Solid Edge part; units mm, degrees
sketch "Sketch1" plane through (0, 0, 0) normal (0, -1, 0) x (1, 0, 0)
  circle A0 centre (0, 0) radius 30.25
extrude "Protrusion1" add sketch "Sketch1" against normal blind 2
sketch "Sketch2" plane through (0, 0, 0) normal (0, -1, 0) x (1, 0, 0)
  circle A0 centre (0, 0) radius 4.5
extrude "Cutout1" cut sketch "Sketch2" against normal through all
sketch "Sketch3" plane through (0, 0, 0) normal (0, -1, 0) x (1, 0, 0)
  circle A0 centre (0, 24) radius 1.5
extrude "Cutout2" cut sketch "Sketch3" against normal through all
pattern_circular "Pattern1" count 4 over 360 about axis through (0, 0, 0) along (0, 1, 0) of "Cutout2"
Source: CAD feature listing. Evaluate the final solid. Frame: model axes, mm. Round coordinates to 2 decimals unless told otherwise and drop trailing zeros. Write each loop counter-clockwise with the first axis right and the second up, starting at its lowest first coordinate (ties: lowest second). Pieces come first, ordered by that corner, then holes. Notation, with made-up numbers: M 14.25,60 L 29.25,60 A10 cw 29.25,65 Z; hole C 68,4 d7. An arc over 180 degrees is marked long. One line per item, written item: value. Start each with the question number.
Item 1: Section query C-C (x = 24). Return the cut outline in (y, z).
Item 2: Section query B-B (z = 3). Return the cut outline in (x, y).
Item 3: Section query D-D (y = 0.85). Return the cut outline in (x, z), plus the area to 3 significant figures.
Item 4: Pin query (flat end, axial travel): pin 1 (5 mm diameter, centred on x = 0, z = 24, fed in from -Y); pin 2 (1 mm diameter, centred on y = 1.5, z = 15.5, fed in from +X). Return the tip coordinate at first contact, or that it passes through.
Item 5: Mould query, pull axis X, two halves, no side actions, for faces 1 (the flat face through (0, 2, -6)), 2 (the cylindrical face through (-0.59, 0.99, 4.46)), 3 (the cylindrical face through (-25.487, 0.986, -0.195)), 4 (the cylindrical face through (-6.56, 0.99, -29.53)). Classes: pulls with the +X half, pulls with the -X half, needs draft (parallel to the pull), parting line crosses it, or undercut.
Item 6: Section query A-A (x = 0). Return the cut outline in (y, z).
Item 7: Ray query, L1, parallel to Z at x = 0, y = 0.9; L2, parallel to Z at x = -24, y = 0.95; L3, parallel to X at y = 1.05, z = 25. Return the intervals inside material, ascending. Write a range as from..to.
Result set:
1. outline: M 0,-18.41 L 2,-18.41 L 2,-1.5 L 0,-1.5 Z; M 0,1.5 L 2,1.5 L 2,18.41 L 0,18.41 Z
2. outline: M -30.1,0 L -3.35,0 L -3.35,2 L -30.1,2 Z; M 3.35,0 L 30.1,0 L 30.1,2 L 3.35,2 Z
3. outline: C 0,0 d60.5; hole C -24,0 d3; hole C 0,0 d9; hole C 0,-24 d3; hole C 0,24 d3; hole C 24,0 d3
3. area: 2,780 mm²
4. pin 1: stops at y = 0
4. pin 2: stops at x = 26.27
5. face 1: needs draft
5. face 2: undercut
5. face 3: undercut
5. face 4: parting line crosses it
6. outline: M 0,-30.25 L 2,-30.25 L 2,-25.5 L 0,-25.5 Z; M 0,-22.5 L 2,-22.5 L 2,-4.5 L 0,-4.5 Z; M 0,4.5 L 2,4.5 L 2,22.5 L 0,22.5 Z; M 0,25.5 L 2,25.5 L 2,30.25 L 0,30.25 Z
7. L1: z = -30.25..-25.5, -22.5..-4.5, 4.5..22.5, 25.5..30.25
7. L2: z = -18.41..-1.5, 1.5..18.41
7. L3: x = -17.03..-1.12, 1.12..17.03
